```python
from build123d import *

# Parameters (mm, degrees)
CYLINDER005_W     = 1.75
CYLINDER005_H     = 3.4
CYLINDER005_ANGLE = 180
CYLINDER004_W     = 1.75
CYLINDER004_H     = 3.4
CYLINDER004_ANGLE = 180
BOX010_W          = 6.5
BOX010_H          = 3.9
BOX010_DEPTH      = 0.2
CYLINDER006_W     = 1.95
CYLINDER006_H     = 0.2
CYLINDER006_ANGLE = 180
CYLINDER007_W     = 1.95
CYLINDER007_H     = 0.2
CYLINDER007_ANGLE = 180
BOX009_W          = 6.5
BOX009_H          = 3.5
BOX009_DEPTH      = 3.4
FILLET001_R       = 0.2


with BuildPart() as cylinder005:
    # Cylinder005 → Cylinder005 (revolve)
    with BuildSketch(Plane(origin=(3.25, 0, 0.6), x_dir=(0, -1, 0), z_dir=(-1, 0, 0))):
        with Locations((0.875, 1.7)):
            Rectangle(CYLINDER005_W, CYLINDER005_H)
    revolve(axis=Axis((3.25, 0, 0.6), (0, 0, 1)), revolution_arc=CYLINDER005_ANGLE)


with BuildPart() as cylinder004:
    # Cylinder004 → Cylinder004 (revolve)
    with BuildSketch(Plane(origin=(-3.25, 0, 0.6), x_dir=(0, 1, 0), z_dir=(1, 0, 0))):
        with Locations((0.875, 1.7)):
            Rectangle(CYLINDER004_W, CYLINDER004_H)
    revolve(axis=Axis((-3.25, 0, 0.6), (0, 0, 1)), revolution_arc=CYLINDER004_ANGLE)


with BuildPart() as cube008:
    # Box010 → Box010 (new body)
    with BuildSketch(Plane(origin=(-3.25, -1.95, 0.4), x_dir=(1, 0, 0), z_dir=(0, 0, 1))):
        with Locations((3.25, 1.95)):
            Rectangle(BOX010_W, BOX010_H)
    extrude(amount=BOX010_DEPTH)


with BuildPart() as cylinder006:
    # Cylinder006 → Cylinder006 (revolve)
    with BuildSketch(Plane(origin=(-3.25, 0, 0.4), x_dir=(0, 1, 0), z_dir=(1, 0, 0))):
        with Locations((0.975, 0.1)):
            Rectangle(CYLINDER006_W, CYLINDER006_H)
    revolve(axis=Axis((-3.25, 0, 0.4), (0, 0, 1)), revolution_arc=CYLINDER006_ANGLE)


with BuildPart() as cylinder007:
    # Cylinder007 → Cylinder007 (revolve)
    with BuildSketch(Plane(origin=(3.25, 0, 0.4), x_dir=(0, -1, 0), z_dir=(-1, 0, 0))):
        with Locations((0.975, 0.1)):
            Rectangle(CYLINDER007_W, CYLINDER007_H)
    revolve(axis=Axis((3.25, 0, 0.4), (0, 0, 1)), revolution_arc=CYLINDER007_ANGLE)


with BuildPart() as cap:
    # Box009 → Box009 (new body)
    with BuildSketch(Plane(origin=(-3.25, -1.75, 0.6), x_dir=(1, 0, 0), z_dir=(0, 0, 1))):
        with Locations((3.25, 1.75)):
            Rectangle(BOX009_W, BOX009_H)
    extrude(amount=BOX009_DEPTH)

    # Fusion001: union Cylinder005, Cylinder004, Cube008, Cylinder006, Cylinder007
    add(cylinder005.part)
    add(cylinder004.part)
    add(cube008.part)
    add(cylinder006.part)
    add(cylinder007.part)

    # Fillet001
    fillet001_edges = [cap.edges().sort_by_distance(p)[0] for p in [
        (0, -1.75, 4),
        (5, 0, 4),
        (0, 1.75, 4),
        (-5, 0, 4),
    ]]
    fillet(fillet001_edges, radius=FILLET001_R)


solid = cap.part
```
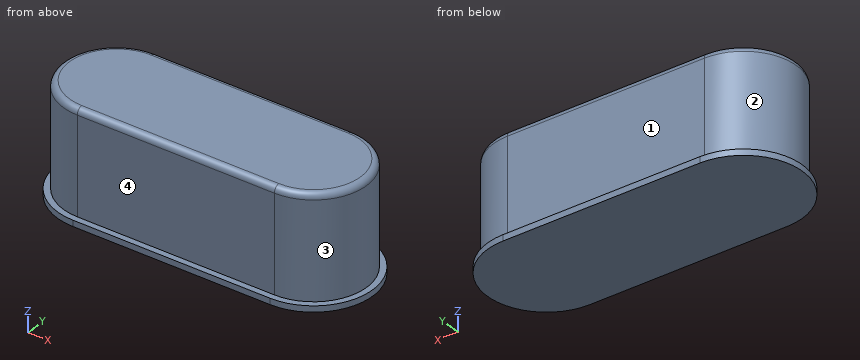
Input: part model. Units: mm. Frame: model coordinates. Face numbers are marked on the shaded views. A direction names the side the tool comes from. Coordinates: 2 decimals unless noted, no trailing zeros. Order: outer loops, then holes, each group sorted by start corner. A loop starts at its lowest first (then second) coordinate and runs counter-clockwise, first axis right, second up. Notation, with made-up numbers: (32.5, 72) - (71.5, 72) arc R18 ccw to (71.5, 106) - close; hole circle Ø10 at (-15.75, 89). An arc over 180 degrees is marked (long way). Return JSON: item names as keys, results as strings.
Q1. First-contact query: pin 1 (1.5 mm diameter, centred on y = -0.5, z = 3, fed in from -X). Flat tip, straight axial feed; report the tip coordinate or a pass-through.
The answers:
{"pin 1": "stops at x = -5"}
Q2. Ray query, probe 1 along Y at (x, z) = (1.25, 2.95); probe 2 along X at (y, z) = (-0.05, 3.55); probe 3 along X at (y, z) = (0.8, 3.6). Return the intervals inside material, ascending.
The answers:
{"probe 1": "y = -1.75 to 1.75", "probe 2": "x = -5 to 5", "probe 3": "x = -4.81 to 4.81"}
Q3. Cut plane B-B (y = 0). Return loops of the section in (x, z).
The answers:
{"outline": "(-5.2, 0.4) - (5.2, 0.4) - (5.2, 0.6) - (5, 0.6) - (5, 3.8) arc R0.2 ccw to (4.8, 4) - (-4.8, 4) arc R0.2 ccw to (-5, 3.8) - (-5, 0.6) - (-5.2, 0.6) - close"}
Q4. Cut plane A-A (x = 1.75). Return loops of the section in (y, z).
The answers:
{"outline": "(-1.95, 0.4) - (1.95, 0.4) - (1.95, 0.6) - (1.75, 0.6) - (1.75, 3.8) arc R0.2 ccw to (1.55, 4) - (-1.55, 4) arc R0.2 ccw to (-1.75, 3.8) - (-1.75, 0.6) - (-1.95, 0.6) - close"}
Q5. Access query for the marked faces 1, 2, 3 and 4. Directions: +Z, -Z, +X, -X, +Y, -Y. A direction counts if a zero-diameter tool reaches every point of the face in a straight line with its end or side. Return the directions, or none.
The answers:
{"face 1": "+Z, +X, -X, +Y", "face 2": "+Z, -X", "face 3": "+Z, +X", "face 4": "+Z, +X, -X, -Y"}
Q6. Cut plane C-C (z = 0.8). Return loops of the section in (x, y).
The answers:
{"outline": "(-3.25, -1.75) - (3.25, -1.75) arc R1.75 ccw to (3.25, 1.75) - (-3.25, 1.75) arc R1.75 ccw to start"}
